from build123d import *

# Parameters (mm, degrees)
SKETCH1_W           = 127
SKETCH1_H           = 76.2
SKETCH1_R           = 4
BOSS_EXTRUDE1_DEPTH = 1.5875


with BuildPart() as part:
    # Sketch1 → Boss-Extrude1 (new body)
    with BuildSketch(Plane.XY):
        with Locations((63.5, 38.1)):
            Rectangle(SKETCH1_W, SKETCH1_H)
        with Locations((76.2, 38.1)):
            Circle(SKETCH1_R, mode=Mode.SUBTRACT)
        with BuildLine():
            Line((38.1, 50.8), (49.2125, 50.8))
            Line((49.2125, 50.8), (49.2125, 25.4))
            Line((49.2125, 25.4), (38.1, 25.4))
            ThreePointArc((38.1, 25.4), (25.4, 38.1), (38.1, 50.8))
        make_face(mode=Mode.SUBTRACT)
        with BuildLine():
            Line((88.9, 25.4), (77.7875, 25.4))
            Line((77.7875, 25.4), (77.7875, 31.10282423))
            ThreePointArc((77.7875, 31.10282423), (83.375, 38.1), (77.7875, 45.09717577))
            Line((77.7875, 45.09717577), (77.7875, 50.8))
            Line((77.7875, 50.8), (88.9, 50.8))
            ThreePointArc((88.9, 50.8), (101.6, 38.1), (88.9, 25.4))
        make_face(mode=Mode.SUBTRACT)
        with BuildLine():
            Line((52.3875, 50.8), (74.6125, 50.8))
            Line((74.6125, 50.8), (74.6125, 45.09717577))
            ThreePointArc((74.6125, 45.09717577), (69.025, 38.1), (74.6125, 31.10282423))
            Line((74.6125, 31.10282423), (74.6125, 25.4))
            Line((74.6125, 25.4), (52.3875, 25.4))
            Line((52.3875, 25.4), (52.3875, 50.8))
        make_face(mode=Mode.SUBTRACT)
    extrude(amount=BOSS_EXTRUDE1_DEPTH)


solid = part.part
Design review of the part built by this model. Coordinates are the model's own, in mm. A direction names the side the tool comes from. Give positions to 0.01 mm unless a question says otherwise; leave off trailing zeros. Loops run counter-clockwise (first coordinate to the right, second up) from the corner with the lowest first, then second, coordinate; pieces in that order, holes last. Notation, with made-up numbers: (9, 17) -> (50, 17) arc R14 cw to (50, 30) -> close; hole circle Ø1 at (-7.75, -19). An arc over 180 degrees is marked (long way). One line per question, with ' | ' between items. Start each with the question number.
(1) For line 1 (Y direction, x = 76.2, z = 0.9); line 2 (X direction, y = 37, z = 0.85); line 3 (Y direction, x = 42.5, z = 0.45), list the stretches that pass through material, from the lowest coordinate up.
(2) We need section A-A (y = 38.1). State the section outline as (x, z) points (1 decimal), and give its area (3 significant figures).
(3) For faces 1 (the face through (77, 47, 0)), 2 (the face through (25.403, 37.821, 0.783)), list the 3-axis set-ups (+Z, -Z, +X, -X, +Y, -Y) from which the entire face can be reached by the end or side of a thin tool; tool diameter is ignored.
(4) We need section D-D (x = 76.2). State the section outline as (y, z) points, and give its area (3 significant figures).
(5) Insertion check: P1, Ø0.8, axis at y = 38.5, z = 1, coming from the -X side. The pin has a flat end and moves straight along its axis. Give the tip position at first contact, or say it passes through.
(6) We need section C-C (z = 0.3). State how many separate pieces and enclosed holes the cut face has, and give its area (3 significant figures).
(7) We need section B-B (x = 62). State the section outline as (y, z) points, and give its area (3 significant figures).
(8) Draft analysis for pull direction X (two halves, no side actions). For faces 3 (the face through (80.015, 39.301, 0.783)), 4 (the face through (77, 47, 1.588)), state which applies: +X half, -X half, draft (parallel to the pull), parting line (faces both ways), or undercut.
The answers:
1) line 1: y = 0 to 34.1, 42.1 to 76.2 | line 2: x = 0 to 25.45, 49.21 to 52.39, 69.11 to 72.35, 80.05 to 83.29, 101.55 to 127 | line 3: y = 0 to 25.4, 50.8 to 76.2
2) outline: (0, 0) -> (25.4, 0) -> (25.4, 1.6) -> (0, 1.6) -> close; (49.2, 0) -> (52.4, 0) -> (52.4, 1.6) -> (49.2, 1.6) -> close; (69, 0) -> (72.2, 0) -> (72.2, 1.6) -> (69, 1.6) -> close; (80.2, 0) -> (83.4, 0) -> (83.4, 1.6) -> (80.2, 1.6) -> close; (101.6, 0) -> (127, 0) -> (127, 1.6) -> (101.6, 1.6) -> close | area: 95.8 mm^2
3) face 1: -Z, +X, -X, +Y, -Y | face 2: +Z, -Z
4) outline: (0, 0) -> (34.1, 0) -> (34.1, 1.59) -> (0, 1.59) -> close; (42.1, 0) -> (76.2, 0) -> (76.2, 1.59) -> (42.1, 1.59) -> close | area: 108 mm^2
5) P1: stops at x = 0
6) separate pieces: 1 | enclosed holes: 4 | area: 8,110 mm^2
7) outline: (0, 0) -> (25.4, 0) -> (25.4, 1.59) -> (0, 1.59) -> close; (50.8, 0) -> (76.2, 0) -> (76.2, 1.59) -> (50.8, 1.59) -> close | area: 80.6 mm^2
8) face 3: undercut | face 4: draft
